Check sheet for the modelled part. Datum: model origin and axes. Units: mm. Give positions to 0.01 mm unless a question says otherwise; leave off trailing zeros. Order: outer loops, then holes, each group sorted by start corner. A loop starts at its lowest first (then second) coordinate and runs counter-clockwise, first axis right, second up.
Item 1: Material ranges on line 1 along Z through (x, y) = (-137, 76); line 2 along Y through (x, z) = (-188, 525.5); line 3 along Z through (x, y) = (-24, 47), recorded low to high.
Item 2: Gauge pin test, flat ends, axial feed: P1, Ø3, axis at x = -97, y = 53, coming from the +Z side; P2, Ø6, axis at x = -294, y = 105, coming from the +Z side. Record the tip position at first contact, or that the pin passes through.
Item 3: Sectioned sample at B-B on y = 50. Record the boundary of the cut face in (x, z), and give its area (3 significant figures).
Item 4: Sectioned sample at C-C on y = 169. Record the boundary of the cut face in (x, z), and give its area (3 significant figures).
from build123d import *

# Parameters (mm, degrees)
F0_W     = 228.6
F0_H     = 558.8
F1_DEPTH = 482.6
F2_SIZE2 = 101.59999
F2_SIZE  = 228.59999


# Not quite as in the source:
# - a fillet or chamfer is up to 0.001 mm smaller than in the source, because OpenCascade refuses the exact size


with BuildPart() as f1:
    # F0 (on Right) → F1 (new body)
    with BuildSketch(Plane.YZ):
        with Locations((114.3, 279.4)):
            Rectangle(F0_W, F0_H)
    extrude(amount=-F1_DEPTH)

    # F2 (size 228.6 and 101.6 in the source; OpenCascade refuses exactly that, so slightly less here)
    f2_edges = [f1.edges().sort_by_distance(p)[0] for p in [
        (-241.3, 0, 558.8),
    ]]
    f2_side = f1.faces().sort_by_distance((-241.3, 114.3, 558.8))[0]
    chamfer(f2_edges, length=F2_SIZE, length2=F2_SIZE2, reference=f2_side)


solid = f1.part
Report:
1. line 1: z = 0 to 490.98
1. line 2: y = 153.67 to 228.6
1. line 3: z = 0 to 478.09
2. P1: stops at z = 481.42
2. P2: stops at z = 505.2
3. outline: (-482.6, 0) - (0, 0) - (0, 479.42) - (-482.6, 479.42) - close
3. area: 231,000 mm2
4. outline: (-482.6, 0) - (0, 0) - (0, 532.31) - (-482.6, 532.31) - close
4. area: 257,000 mm2
